```python
from build123d import *

# Parameters (mm, degrees)
SKETCH1_R           = 12.5
BOSS_EXTRUDE1_DEPTH = 2.65
BOSS_EXTRUDE2_DEPTH = 2.65
CIRPATTERN1_COUNT   = 37
CUT_EXTRUDE1_DEPTH  = 6
SKETCH5_W           = 7.2
SKETCH5_H           = 20
BOSS_EXTRUDE3_DEPTH = 2.65
FILLET1_R           = 2.5
SKETCH6_R           = 1.755
CUT_EXTRUDE2_DEPTH  = 36.020633077
SKETCH7_R           = 1.75
CUT_EXTRUDE3_DEPTH  = 36.020633077


with BuildPart() as part:
    # Sketch1 → Boss-Extrude1 (new body)
    with BuildSketch(Plane.XY):
        Circle(SKETCH1_R)
    extrude(amount=BOSS_EXTRUDE1_DEPTH)

    # Sketch2 → Boss-Extrude2 (add)
    with BuildSketch(Plane.XY.offset(2.65)):
        with BuildLine():
            Line((-1.490008762, 12.410877241), (-0.647496991, 12.483218641))
            ThreePointArc((-0.647496991, 12.483218641), (-0.560389102, 13.376964625), (-0.786565642, 14.245995027))
            ThreePointArc((-0.786565642, 14.245995027), (-1.294727869, 14.469274157), (-1.768283344, 14.179744139))
            ThreePointArc((-1.768283344, 14.179744139), (-1.872233227, 13.257068705), (-1.490008762, 12.410877241))
        make_face()
    boss_extrude2 = extrude(amount=-BOSS_EXTRUDE2_DEPTH)

    # CirPattern1: Boss-Extrude2 ×37 about axis
    cirpattern1_axis = Axis((-0.005621408, 0.062130421, 0), (0, 0, 1))
    for i in range(1, CIRPATTERN1_COUNT):
        add(boss_extrude2.rotate(cirpattern1_axis, i * 360 / CIRPATTERN1_COUNT))

    # Sketch3 → Cut-Extrude1 (cut)
    with BuildSketch(Plane.XY.offset(2.65)):
        with BuildLine():
            ThreePointArc((2.617339204, -12.222910271), (12.455404486, -0.045944124), (2.707439802, 12.203268813))
            ThreePointArc((2.707439802, 12.203268813), (2.478611131, 13.53676799), (3.259731136, 14.641500607))
            ThreePointArc((3.259731136, 14.641500607), (14.955387478, -0.055165786), (3.151627992, -14.665150122))
            ThreePointArc((3.151627992, -14.665150122), (3.390288032, -13.333375366), (2.617339204, -12.222910271))
        make_face()
    extrude(amount=-CUT_EXTRUDE1_DEPTH, mode=Mode.SUBTRACT)

    # Sketch5 → Boss-Extrude3 (add)
    with BuildSketch(Plane.XY.offset(2.65)):
        with Locations((-0.55815824, 21.788117748)):
            Rectangle(SKETCH5_W, SKETCH5_H)
    extrude(amount=-BOSS_EXTRUDE3_DEPTH)

    # Fillet1
    fillet1_edges = [part.edges().sort_by_distance(p)[0] for p in [
        (3.04184176, 31.788117748, 1.325),
        (-4.15815824, 31.788117748, 1.325),
    ]]
    fillet(fillet1_edges, radius=FILLET1_R)

    # Sketch6 → Cut-Extrude2 (cut, through all)
    with BuildSketch(Plane.XY.offset(2.65)):
        Circle(SKETCH6_R)
    extrude(amount=-CUT_EXTRUDE2_DEPTH, mode=Mode.SUBTRACT)

    # Sketch7 → Cut-Extrude3 (cut, through all)
    with BuildSketch(Plane.XY.offset(2.65)):
        with Locations((-0.612089544, 28.238117748)):
            Circle(SKETCH7_R)
    extrude(amount=-CUT_EXTRUDE3_DEPTH, mode=Mode.SUBTRACT)


solid = part.part
```
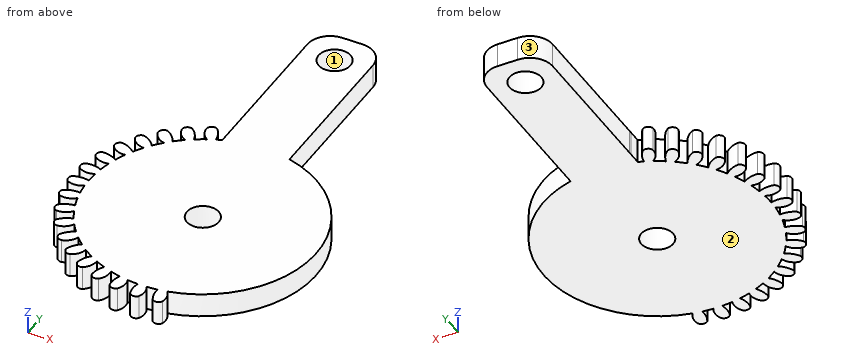
The model under review builds one solid part; all positions refer to its coordinate system, in mm. Face numbers are marked on the shaded views. Round coordinates to 2 decimals unless told otherwise and drop trailing zeros. Order: outer loops, then holes, each group sorted by start corner. A loop starts at its lowest first (then second) coordinate and runs counter-clockwise, first axis right, second up.
(1) For P1, Ø0.8, axis at y = 23.5, z = 1.5, coming from the -X side; P2, Ø1.5, axis at y = 12.5, z = 1.5, coming from the -X side, all flat-tipped, find the tip position at first contact; note any pin that passes through.
Working result:
P1: stops at x = -4.16
P2: stops at x = -8.38
(2) Take a section at C-C, the plane x = 7.5. State the section outline as (y, z) points.
Working result:
outline: (-9.97, 0) - (9.97, 0) - (9.97, 2.65) - (-9.97, 2.65) - close
(3) Wall thickness on L1, parallel to Y at x = 0, z = 1.5 (3 decimals); L2, parallel to Y at x = -10, z = 1.3; L3, parallel to X at y = 15.5, z = 1.95: over which ranges is each line inside the solid? List them lowest first.
Working result:
L1: y = -14.399 to -1.755, 1.755 to 26.599, 29.878 to 31.788
L2: y = -9.64 to -8.03, -7.5 to 8.11, 9.44 to 10.51
L3: x = -4.16 to 3.04
(4) Mouldability with a two-part tool opening along X and no side actions: class the marked faces 1, 2 and 3 as released by +X, released by -X, zero draft, split by the parting line, or undercut.
Working result:
face 1: undercut
face 2: zero draft
face 3: released by -X
(5) Take a section at D-D, the plane z = 1. Count the separate pieces of the cut face and the enclosed holes in it, plus the area to 3 significant figures.
Working result:
separate pieces: 1
enclosed holes: 2
area: 648 mm2
(6) Take a section at B-B, the plane y = 19. State the section outline as (x, z) points.
Working result:
outline: (-4.16, 0) - (3.04, 0) - (3.04, 2.65) - (-4.16, 2.65) - close
(7) Take a section at A-A, the plane x = 0. State the section outline as (y, z) points (3 decimals).
Working result:
outline: (-14.399, 0) - (-1.755, 0) - (-1.755, 2.65) - (-14.399, 2.65) - close; (1.755, 0) - (26.599, 0) - (26.599, 2.65) - (1.755, 2.65) - close; (29.878, 0) - (31.788, 0) - (31.788, 2.65) - (29.878, 2.65) - close
